Could you check a few things on this model? Use its own coordinates, in mm. Face numbers are marked on the shaded views. A direction names the side the tool comes from. Round coordinates to 2 decimals unless told otherwise and drop trailing zeros. Write each loop counter-clockwise with the first axis right and the second up, starting at its lowest first coordinate (ties: lowest second). Pieces come first, ordered by that corner, then holes. Notation, with made-up numbers: (-8.75, 5.5) - (32.25, 5.5) arc R29 cw to (32.25, 35.5) - close; hole circle Ø8 at (27, 8.25). An arc over 180 degrees is marked (long way). Write each question's results on one line, items separated by ' | '. Start each with the question number.
(1) Imagine slicing it at C-C on x = 3.75. Write out the boundary of the cut face in (y, z).
(2) On a 3-axis mill with a long thin cutter (end or side, diameter ignored), from which of +Z, -Z, +X, -X, +Y, -Y can I reach the whole of each face in a straight line? I mean the marked faces 1 and 2. Say none if no direction works.
(3) Imagine slicing it at A-A on z = 0. Write out the boundary of the cut face in (x, y) (3 decimals), then the cut area to 3 significant figures.
(4) For P1, Ø8, axis at x = 3.5, y = 3, coming from the +Z side; P2, Ø3, axis at x = 7, z = 2.5, coming from the -Y side; P3, Ø1.5, axis at x = 9, y = 5, coming from the +Z side; P4, Ø4, axis at x = 3.5, y = 3.5, coming from the -Z side, each with a flat end and sliding along its axis, tell me the tip position at first contact or that it passes through.
(5) Thinking about a two-plate mould opening in Y: for the marked faces 3, 4 and 5, which applies, +Y half, -Y half, draft (parallel to the pull), parting line (faces both ways), or undercut?
(6) Please list where these lines run through material, in increasing order: line 1 (Y direction, x = 9.25, z = 0); line 2 (Y direction, x = 13, z = -3); line 3 (Z direction, x = 6.5, y = -1). Write a range as [from, to].
```python
from build123d import *

# Parameters (mm, degrees)
SKETCH1_R           = 7.62
SKETCH1_W           = 6.604
SKETCH1_H           = 6.604
BOSS_EXTRUDE1_DEPTH = 18.415
FILLET1_R           = 0.635


with BuildPart() as part:
    # Sketch1 → Boss-Extrude1 (new body)
    with BuildSketch(Plane(origin=(0, 0, 0), x_dir=(0, 0, -1), z_dir=(1, 0, 0))):
        Circle(SKETCH1_R)
        Rectangle(SKETCH1_W, SKETCH1_H, mode=Mode.SUBTRACT)
    extrude(amount=BOSS_EXTRUDE1_DEPTH)

    # Fillet1
    fillet1_edges = [part.edges().sort_by_distance(p)[0] for p in [
        (18.415, 0, 3.302),
        (18.415, -3.302, 0),
        (0, 0, 7.62),
        (18.415, 0, 7.62),
        (0, 0, -3.302),
        (0, 3.302, 0),
        (0, 0, 3.302),
        (0, -3.302, 0),
        (18.415, 0, -3.302),
        (18.415, 3.302, 0),
    ]]
    fillet(fillet1_edges, radius=FILLET1_R)


solid = part.part
```
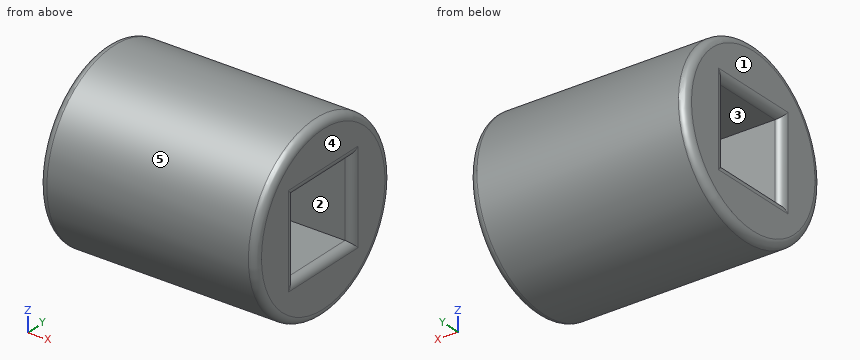
Response:
1) outline: circle Ø15.24 at (0, 0); hole (-3.3, -3.3) - (3.3, -3.3) - (3.3, 3.3) - (-3.3, 3.3) - close
2) face 1: +Z, -Z, -X, +Y, -Y | face 2: +X, -X
3) outline: (0, -6.985) arc R0.635 ccw to (0.635, -7.62) - (17.78, -7.62) arc R0.635 ccw to (18.415, -6.985) - (18.415, -3.937) arc R0.635 ccw to (17.78, -3.302) - (0.635, -3.302) arc R0.635 ccw to (0, -3.937) - close; (0, 3.937) arc R0.635 ccw to (0.635, 3.302) - (17.78, 3.302) arc R0.635 ccw to (18.415, 3.937) - (18.415, 6.985) arc R0.635 ccw to (17.78, 7.62) - (0.635, 7.62) arc R0.635 ccw to (0, 6.985) - close | area: 158 mm²
4) P1: z = 7.62 | P2: y = -7.55 | P3: z = 6.32 | P4: z = -7.47
5) face 3: undercut | face 4: draft | face 5: parting line
6) line 1: [-7.62, -3.3], [3.3, 7.62] | line 2: [-7, -3.3], [3.3, 7] | line 3: [-7.55, -3.3], [3.3, 7.55]
